from build123d import *

# Parameters (mm, degrees)
F0_W           = 9
F0_H           = 6.5
F1_DEPTH       = 300
F3_D           = 3.5
F3_CBORE_D     = 6
F3_CBORE_DEPTH = 4.5


with BuildPart() as f1:
    # F0 (on Front) → F1 (new body)
    with BuildSketch(Plane.XZ):
        with Locations((4.5, 3.25)):
            Rectangle(F0_W, F0_H)
    extrude(amount=F1_DEPTH)

    # F3 (through all)
    with Locations(Plane.XY.offset(6.5)):
        with Locations((4.5, -292.5), (4.5, -272.5), (4.5, -252.5), (4.5, -232.5), (4.5, -212.5), (4.5, -192.5), (4.5, -172.5), (4.5, -152.5), (4.5, -132.5), (4.5, -112.5), (4.5, -92.5), (4.5, -72.5), (4.5, -52.5), (4.5, -32.5), (4.5, -12.5)):
            CounterBoreHole(F3_D / 2, F3_CBORE_D / 2, F3_CBORE_DEPTH)


solid = f1.part
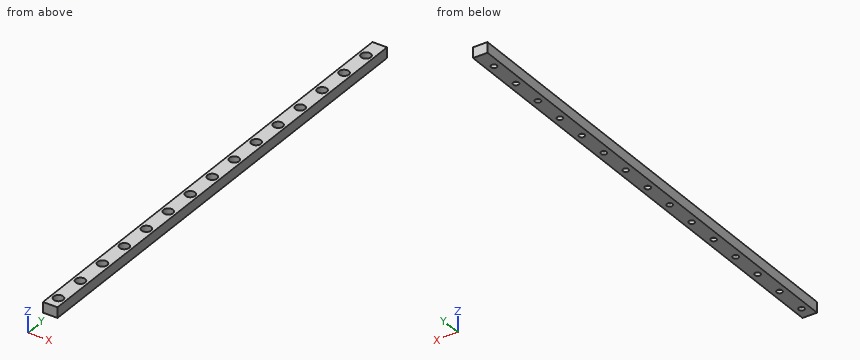
Work out the finished part from the listing and answer in its coordinate system (mm). Give positions to 0.01 mm unless a question says otherwise; leave off trailing zeros. Use a Markdown table: item, result. Add a question column.
1. Find the intervals of material crossed by probe 1 along X at (y, z) = (-92.5, 1.3); probe 2 along X at (y, z) = (-172.5, 5.25); probe 3 along Z at (x, y) = (2, -132.5), in increasing order.
2. Section A-A on z = 4.75 is taken. State how many separate pieces and enclosed holes the cut face has, and give its area (3 significant figures).
3. Flat-ended cylindrical pins translate along their axes: pin 1 Ø3 at (x, y) = (4.5, -132.5) entering from -Z; pin 2 Ø4.5 at (x, y) = (4.5, -292.5) entering from +Z. Find the tip coordinate at first contact, or state that the pin passes through.
Results below:
| question | item | result |
|---|---|---|
| 1 | probe 1 | x = 0 to 2.75, 6.25 to 9 |
| 1 | probe 2 | x = 0 to 1.5, 7.5 to 9 |
| 1 | probe 3 | z = 0 to 2 |
| 2 | separate pieces | 1 |
| 2 | enclosed holes | 15 |
| 2 | area | 2,280 mm^2 |
| 3 | pin 1 | passes through |
| 3 | pin 2 | stops at z = 2 |
